```python
from build123d import *

# Parameters (mm, degrees)
SKETCH_1_W          = 2
SKETCH_1_H          = 50
EXTRUDE_1_DEPTH     = 2
SKETCH_3_W          = 50
SKETCH_3_H          = 20
EXTRUDE_3_DEPTH     = 20
SKETCH_4_W          = 10
SKETCH_4_H          = 11
CUT_EXTRUDE_1_DEPTH = 58.801384066
SKETCH_6_W          = 15
SKETCH_6_H          = 20
EXTRUDE_4_DEPTH     = 5
SKETCH_7_W          = 3
SKETCH_7_H          = 80
CUT_EXTRUDE_4_DEPTH = 50.406477308
SKETCH_8_R          = 1.1
CUT_EXTRUDE_5_DEPTH = 49.590122453
SKETCH_9_R          = 0.8
CUT_EXTRUDE_6_DEPTH = 2


with BuildPart() as part:
    # 草图1 → 凸台-拉伸1 (new body)
    with BuildSketch(Plane(origin=(0, 0, 0), x_dir=(1, 0, 0), z_dir=(0, 1, 0))):
        Rectangle(SKETCH_1_W, SKETCH_1_H)
    extrude(amount=EXTRUDE_1_DEPTH)

    # 草图3 → 凸台-拉伸3 (add)
    with BuildSketch(Plane(origin=(1, 0, 0), x_dir=(0, 0, -1), z_dir=(1, 0, 0))):
        with Locations((0, 10)):
            Rectangle(SKETCH_3_W, SKETCH_3_H)
    extrude(amount=EXTRUDE_3_DEPTH)

    # 草图4 → 切除-拉伸1 (cut, through all)
    with BuildSketch(Plane.XY.offset(25)):
        with Locations((6, 14.5)):
            Rectangle(SKETCH_4_W, SKETCH_4_H)
    extrude(amount=-CUT_EXTRUDE_1_DEPTH, mode=Mode.SUBTRACT)

    # 草图6 → 凸台-拉伸4 (add)
    with BuildSketch(Plane(origin=(21, 0, 0), x_dir=(0, 0, -1), z_dir=(1, 0, 0))):
        with Locations((-32.5, 10)):
            Rectangle(SKETCH_6_W, SKETCH_6_H)
        with Locations((32.5, 10)):
            Rectangle(SKETCH_6_W, SKETCH_6_H)
    extrude(amount=-EXTRUDE_4_DEPTH)

    # 草图7 → 切除-拉伸4 (cut, through all)
    with BuildSketch(Plane(origin=(0, 20, 0), x_dir=(1, 0, 0), z_dir=(0, 1, 0))):
        with Locations((19.5, 0)):
            Rectangle(SKETCH_7_W, SKETCH_7_H)
    extrude(amount=-CUT_EXTRUDE_4_DEPTH, mode=Mode.SUBTRACT)

    # 草图8 → 切除-拉伸5 (cut, through all)
    with BuildSketch(Plane(origin=(18, 0, 0), x_dir=(0, 0, -1), z_dir=(1, 0, 0))):
        with Locations((30, 15)):
            Circle(SKETCH_8_R)
        with Locations((30, 5)):
            Circle(SKETCH_8_R)
        with Locations((-30, 15)):
            Circle(SKETCH_8_R)
        with Locations((-30, 5)):
            Circle(SKETCH_8_R)
    extrude(amount=-CUT_EXTRUDE_5_DEPTH, mode=Mode.SUBTRACT)

    # 草图9 → 切除-拉伸6 (cut)
    with BuildSketch(Plane(origin=(0, 20, 0), x_dir=(1, 0, 0), z_dir=(0, 1, 0))):
        with Locations(Location((13.5, -17, 0), (0, 0, 270))):
            Circle(SKETCH_9_R)
        with Locations(Location((13.5, 17, 0), (0, 0, 270))):
            Circle(SKETCH_9_R)
    extrude(amount=-CUT_EXTRUDE_6_DEPTH, mode=Mode.SUBTRACT)


solid = part.part
```
The model under review builds one solid part; all positions refer to its coordinate system, in mm. A direction names the side the tool comes from. Round coordinates to 2 decimals unless told otherwise and drop trailing zeros. Order: outer loops, then holes, each group sorted by start corner. A loop starts at its lowest first (then second) coordinate and runs counter-clockwise, first axis right, second up. Notation, with made-up numbers: M 88.5,-36 L 107.5,-36 A27 cw 107.5,-16 Z; hole C -32.5,-19 d11. An arc over 180 degrees is marked long. Use a Markdown table: item, result.
1) Draft analysis for pull direction Y (two halves, no side actions). For faces 1 (the face through (17.01, 5.33, -31.05)), 2 (the face through (11, 14, 0)), 3 (the face through (14, 18, -17)), state which applies: released by +Y, released by -Y, zero draft, split by the parting line, or undercut.
Report:
| item | result |
|---|---|
| face 1 | undercut |
| face 2 | zero draft |
| face 3 | released by +Y |
2) Consider section D-D (z = 8.5). Write out the cut boundary in (x, y), then the cut area to 3 significant figures.
Report:
| item | result |
|---|---|
| outline | M -1,0 L 18,0 L 18,20 L 11,20 L 11,9 L 1,9 L 1,2 L -1,2 Z |
| area | 234 mm^2 |
3) Tool access review of faces 4 (the face through (14.04, 19.01, 16.41)), 5 (the face through (1, 6, 0)), 6 (the face through (9, 8, -25)): name each direction out of +Z, -Z, +X, -X, +Y, -Y from which nothing blocks a thin tool from reaching the whole face with its end or side.
Report:
| item | result |
|---|---|
| face 4 | +Y |
| face 5 | +Z, -Z, -X, +Y |
| face 6 | -Z, -X, +Y, -Y |
4) Insertion check: pin 1 (1.8 mm diameter, centred on x = 13.5, z = 17, fed in from +Y); pin 2 (2 mm diameter, centred on x = 0.5, z = -5, fed in from +Y); pin 3 (4 mm diameter, centred on y = 15.5, z = 22, fed in from -X); pin 4 (12 mm diameter, centred on y = 11.5, z = -26, fed in from -X). Each pin has a flat end and moves straight along its axis. Give the tip position at first contact, or say it passes through.
Report:
| item | result |
|---|---|
| pin 1 | y = 20 |
| pin 2 | y = 9 |
| pin 3 | x = 11 |
| pin 4 | x = 1 |
5) Consider section C-C (y = 11.5). Write out the cut boundary in (x, z), then the cut area to 3 significant figures.
Report:
| item | result |
|---|---|
| outline | M 11,-25 L 16,-25 L 16,-40 L 18,-40 L 18,40 L 16,40 L 16,25 L 11,25 Z |
| area | 410 mm^2 |
6) Consider section B-B (z = 30). Write out the cut boundary in (x, y), then the cut area to 3 significant figures.
Report:
| item | result |
|---|---|
| outline | M 16,0 L 18,0 L 18,3.9 L 16,3.9 Z; M 16,6.1 L 18,6.1 L 18,13.9 L 16,13.9 Z; M 16,16.1 L 18,16.1 L 18,20 L 16,20 Z |
| area | 31.2 mm^2 |
7) Wall thickness on line 1 along Y through (x, z) = (17.1, 30); line 2 along X through (y, z) = (18.4, -17); line 3 along Y through (x, z) = (10.25, -17): over which ranges is each line inside the solid? List them lowest first. Write a range as [from, to].
Report:
| item | result |
|---|---|
| line 1 | [0, 3.9], [6.1, 13.9], [16.1, 20] |
| line 2 | [11, 12.7], [14.3, 18] |
| line 3 | [0, 9] |
8) Consider section A-A (y = 15). Write out the cut boundary in (x, z), then the cut area to 3 significant figures.
Report:
| item | result |
|---|---|
| outline | M 11,-25 L 16,-25 L 16,-28.9 L 18,-28.9 L 18,28.9 L 16,28.9 L 16,25 L 11,25 Z; M 16,-40 L 18,-40 L 18,-31.1 L 16,-31.1 Z; M 16,31.1 L 18,31.1 L 18,40 L 16,40 Z |
| area | 401 mm^2 |
